Input: part model. Units: mm. Frame: model coordinates. A direction names the side the tool comes from. Coordinates: 2 decimals unless noted, no trailing zeros. Loops run counter-clockwise (first coordinate to the right, second up) from the corner with the lowest first, then second, coordinate; pieces in that order, holes last.
Item 1: Section A-A on x = -10. Return loops of the section in (y, z).
Item 2: Reachability of faces 1 (the flat face through (-16, 28.757, 4)), 2 (the flat face through (-15.383, 3.189, -0.07)), 3 (the flat face through (-1, 20, 0)) from +Z, -Z, +X, -X, +Y, -Y: full face, straight path, thin tool, end or side. Return the list, or none.
Item 3: Pull-direction query (Z, two-part tool) for faces 4 (the flat face through (4.33, 40.68, 0.06)), 5 (the flat face through (-8, 25.5, 0)), 6 (the flat face through (-16, 35, 2)); classes: released by +Z, released by -Z, zero draft, split by the parting line, or undercut.
Item 4: Ray query, line 1 along Z through (x, y) = (-10, 18.5); line 2 along Y through (x, z) = (-5.5, -2.25); line 3 along Y through (x, z) = (-8, -4.25). Return the intervals inside material, ascending.
Item 5: Contact query for flat-ended pins moving along their axis: P1, Ø3.5, axis at x = -2, z = 4, coming from the -Y side; P2, Ø2.5, axis at y = 35.5, z = -4, coming from the -X side; P3, Ø2.5, axis at x = -3, y = 35.5, coming from the -Z side; P4, Ø2, axis at x = -18, z = 2.5, coming from the +Y side. Output: stop coordinate, or through.
```python
from build123d import *

# Parameters (mm, degrees)
BOSS_EXTRUDE1_DEPTH     = 5
CUT_EXTRUDE1_DEPTH      = 52.295711322
CUT_EXTRUDE1_DEPTH_BACK = 10
CUT_EXTRUDE3_START      = -10
CUT_EXTRUDE3_DEPTH      = 10
CUT_EXTRUDE4_DEPTH      = 52.295711322
CUT_EXTRUDE4_DEPTH_BACK = 10
CUT_EXTRUDE5_DEPTH      = 10
CUT_EXTRUDE6_DEPTH      = 3
SKETCH9_R               = 4
CUT_EXTRUDE7_DEPTH      = 13
CUT_EXTRUDE8_REACH      = 41.4
SKETCH10_R              = 1.75
CUT_EXTRUDE9_DEPTH      = 13
SKETCH12_W              = 6
SKETCH12_H              = 21
CUT_EXTRUDE10_DEPTH     = 4
CUT_EXTRUDE11_DEPTH     = 5.830271703
CHAMFER1_SIZE           = 1


# Read off the part's stored shape, not the designer's step: Cut-Extrude3
with BuildPart() as part:
    # Sketch1 → Boss-Extrude1 (new, symmetric)
    with BuildSketch(Plane.XY):
        Polygon((-22.5, 45), (-22.5, 0), (22.5, 0), (22.5, 26), (3.5, 45), align=None)
    extrude(amount=BOSS_EXTRUDE1_DEPTH, both=True)

    # Sketch2 → Cut-Extrude1 (cut, two sides: drawn at the far end of the back side and taken through both)
    with BuildSketch(Plane.XY.offset(5).offset(-CUT_EXTRUDE1_DEPTH_BACK)):
        with BuildLine():
            Line((-111.960387508, -74.460387508), (-22.5, 15))
            Line((-22.5, 15), (-19.5, 18))
            Line((-19.5, 18), (-19.5, 21.5))
            ThreePointArc((-19.5, 21.5), (-17.9, 23.5), (-19.5, 25.5))
            Line((-19.5, 25.5), (-19.5, 40))
            Line((-19.5, 40), (-14.5, 45))
            Line((-14.5, 45), (74.960387508, 134.460387508))
            Line((74.960387508, 134.460387508), (-113.613392046, 303.176768247))
            Line((-113.613392046, 303.176768247), (-300.534167062, 94.255993231))
            Line((-300.534167062, 94.255993231), (-111.960387508, -74.460387508))
        make_face()
    extrude(amount=CUT_EXTRUDE1_DEPTH + CUT_EXTRUDE1_DEPTH_BACK, mode=Mode.SUBTRACT)

    # Cut-Extrude3 outline → Cut-Extrude3 (cut)
    with BuildSketch(Plane.XY.offset(5).offset(CUT_EXTRUDE3_START)):
        Polygon((21.5, 27), (21.5, 14.5), (22.5, 13.5), (22.5, 26), align=None)
        with BuildLine():
            Line((22.5, 0), (22.5, 3.8))
            ThreePointArc((22.5, 3.8), (21.972792206, 2.527207794), (20.7, 2))
            Line((20.7, 2), (17.5, 2))
            ThreePointArc((17.5, 2), (15.514097811, 3.762950432), (17.029242744, 5.943807502))
            Line((17.029242744, 5.943807502), (18.5, 6.3))
            Line((18.5, 6.3), (18.5, 7))
            Line((18.5, 7), (-16.5, 7))
            Line((-16.5, 7), (-16.5, 5.5))
            Line((-16.5, 5.5), (-15.081081244, 5.5))
            ThreePointArc((-15.081081244, 5.5), (-14.751598645, 5.326806563), (-14.707437165, 4.957206084))
            Line((-14.707437165, 4.957206084), (-16.078389668, 1.369880369))
            ThreePointArc((-16.078389668, 1.369880369), (-16.706486271, 0.552810765), (-17.679866918, 0.214228137))
            Line((-17.679866918, 0.214228137), (-21.455599386, 0.046417805))
            ThreePointArc((-21.455599386, 0.046417805), (-22.191230564, 0.322797329), (-22.5, 1.045431612))
            Line((-22.5, 1.045431612), (-22.5, 0))
            Line((-22.5, 0), (22.5, 0))
        make_face()
    extrude(amount=CUT_EXTRUDE3_DEPTH, mode=Mode.SUBTRACT)

    # Sketch3 → Cut-Extrude4 (cut, two sides: drawn at the far end of the back side and taken through both)
    with BuildSketch(Plane.XY.offset(5).offset(-CUT_EXTRUDE4_DEPTH_BACK)):
        Polygon((85.857284299, 122.40753683), (5.974873734, 42.525126266), (5.621320344, 42.171572875), (20.792893219, 27), (21.146446609, 27.353553391), (101.028857174, 107.235963955), (260.793678303, 267.000785084), (245.622105428, 282.17235796), align=None)
    extrude(amount=CUT_EXTRUDE4_DEPTH + CUT_EXTRUDE4_DEPTH_BACK, mode=Mode.SUBTRACT)

    # Sketch7 → Cut-Extrude5 (cut)
    with BuildSketch(Plane.XY.offset(5)):
        with BuildLine():
            Line((-16.5, 7.7), (-16.5, 11))
            ThreePointArc((-16.5, 11), (-16.153059775, 12.400454865), (-15.192484115, 13.476993646))
            Line((-15.192484115, 13.476993646), (-11.5, 16))
            Line((-11.5, 16), (-4.3, 16))
            ThreePointArc((-4.3, 16), (-3.734314575, 16.234314575), (-3.5, 16.8))
            Line((-3.5, 16.8), (-3.5, 22.2))
            ThreePointArc((-3.5, 22.2), (-3.734314575, 22.765685425), (-4.3, 23))
            Line((-4.3, 23), (-14.25, 23))
            ThreePointArc((-14.25, 23), (-15.5, 24.25), (-14.25, 25.5))
            Line((-14.25, 25.5), (-4.2, 25.5))
            ThreePointArc((-4.2, 25.5), (-1.9372583, 24.5627417), (-1, 22.3))
            Line((-1, 22.3), (-1, 17.183557492))
            ThreePointArc((-1, 17.183557492), (-1.825475903, 15.038415232), (-3.876022072, 14))
            Line((-3.876022072, 14), (-13.702486205, 13))
            ThreePointArc((-13.702486205, 13), (-14.98407756, 12.35099048), (-15.5, 11.010276568))
            Line((-15.5, 11.010276568), (-15.5, 7.9))
            Line((-15.5, 7.9), (-16.5, 7.7))
        make_face()
    extrude(amount=-CUT_EXTRUDE5_DEPTH, mode=Mode.SUBTRACT)

    # Sketch8 → Cut-Extrude6 (cut)
    with BuildSketch(Plane.XY.offset(5)):
        Polygon((-17.5, 20), (-13.5, 20), (-13.5, 17), (-17.5, 15), align=None)
        Polygon((-16.5, 38.757359313), (-16.5, 28.757359313), (-14.5, 28.757359313), (-14.5, 40.757359313), align=None)
        Polygon((0.4, 42), (-4.5, 42), (-4.5, 33.5), (0.4, 38.4), align=None)
        with BuildLine():
            Line((-3.52075849, 10), (18.5, 10))
            Line((18.5, 10), (18.5, 20.807611845))
            Line((18.5, 20.807611845), (16.520101013, 22.787510832))
            Line((16.520101013, 22.787510832), (8.74192642, 15.009336239))
            Line((8.74192642, 15.009336239), (4.145732342, 19.605530317))
            Line((4.145732342, 19.605530317), (11.923906935, 27.38370491))
            Line((11.923906935, 27.38370491), (6.267052685, 33.040559159))
            Line((6.267052685, 33.040559159), (0.045175397, 26.818681871))
            ThreePointArc((0.045175397, 26.818681871), (1.490346539, 24.761697843), (2, 22.3))
            Line((2, 22.3), (2, 17.183557492))
            ThreePointArc((2, 17.183557492), (0.400640437, 13.027344363), (-3.572292764, 11.015414852))
            ThreePointArc((-3.572292764, 11.015414852), (-4.029119362, 10.483214857), (-3.52075849, 10))
        make_face()
    cut_extrude6 = extrude(amount=-CUT_EXTRUDE6_DEPTH, mode=Mode.SUBTRACT)

    # Mirror1: Cut-Extrude6 across plane
    add(cut_extrude6.mirror(Plane.XY), mode=Mode.SUBTRACT)

    # Sketch9 → Cut-Extrude7 (cut)
    with BuildSketch(Plane(origin=(0, 45, 0), x_dir=(1, 0, 0), z_dir=(0, 1, 0))):
        with Locations(Location((-10, 0, 0), (0, 0, 270))):
            Circle(SKETCH9_R)
    extrude(amount=-CUT_EXTRUDE7_DEPTH, mode=Mode.SUBTRACT)

    # Cut-Extrude8: up to this face of the body (flat: up to its plane)
    cut_extrude8_end = Plane(part.part.faces().sort_by_distance((-7.9, 16, 0))[0])
    # Sketch10 → Cut-Extrude8 (cut, up to the picked face)
    with BuildSketch(Plane(origin=(0, 32, 0), x_dir=(1, 0, 0), z_dir=(0, 1, 0)), mode=Mode.PRIVATE) as cut_extrude8_sk1:
        with Locations(Location((-10, 0, 0), (0, 0, 270))):
            Circle(SKETCH10_R)
    cut_extrude8_tool1 = split(extrude(cut_extrude8_sk1.sketch, amount=-CUT_EXTRUDE8_REACH, mode=Mode.PRIVATE), bisect_by=cut_extrude8_end, keep=Keep.BOTH, mode=Mode.PRIVATE)
    add(cut_extrude8_tool1.solids().sort_by(Axis((-10, 32, 0), (0, -1, 0)))[0], mode=Mode.SUBTRACT)

    # Sketch11 → Cut-Extrude9 (cut)
    with BuildSketch(Plane.XY.offset(5)):
        with BuildLine():
            Line((-4.219533003, 31.039254845), (-0.683999097, 27.503720939))
            Line((-0.683999097, 27.503720939), (2.851534809, 31.039254845))
            Line((2.851534809, 31.039254845), (-0.683999097, 34.574788751))
            Line((-0.683999097, 34.574788751), (-2.098212659, 33.160575189))
            ThreePointArc((-2.098212659, 33.160575189), (-2.098212659, 32.453468408), (-2.80531944, 32.453468408))
            Line((-2.80531944, 32.453468408), (-4.219533003, 31.039254845))
        make_face()
        with BuildLine():
            Line((11.336816184, 18.311332784), (9.922602621, 16.897119222))
            Line((9.922602621, 16.897119222), (6.387068715, 20.432653128))
            Line((6.387068715, 20.432653128), (9.922602621, 23.968187033))
            Line((9.922602621, 23.968187033), (13.458136527, 20.432653128))
            Line((13.458136527, 20.432653128), (12.043922965, 19.018439565))
            ThreePointArc((12.043922965, 19.018439565), (11.336816184, 19.018439565), (11.336816184, 18.311332784))
        make_face()
    extrude(amount=-CUT_EXTRUDE9_DEPTH, mode=Mode.SUBTRACT)

    # Sketch12 → Cut-Extrude10 (cut)
    with BuildSketch(Plane(origin=(23.896446609, 23.896446609, 0), x_dir=(0, 0, -1), z_dir=(0.7071067811865471, 0.7071067811865479, 0))):
        with Locations((0, 15.204222165)):
            Rectangle(SKETCH12_W, SKETCH12_H)
    extrude(amount=-CUT_EXTRUDE10_DEPTH, mode=Mode.SUBTRACT)

    # Sketch13 → Cut-Extrude11 (cut)
    with BuildSketch(Plane(origin=(21.068019485, 21.068019485, 0), x_dir=(0, 0, -1), z_dir=(0.7071067811865471, 0.7071067811865479, 0))):
        Polygon((-1.5, 24.931727984), (1.5, 24.931727984), (1.5, 21.431727984), (2.75, 21.431727984), (2.75, 19.931727984), (-2.75, 19.931727984), (-2.75, 21.431727984), (-1.5, 21.431727984), align=None)
        Polygon((-1.5, 5.476716347), (-1.5, 8.976716347), (-2.75, 8.976716347), (-2.75, 10.476716347), (2.75, 10.476716347), (2.75, 8.976716347), (1.5, 8.976716347), (1.5, 5.476716347), align=None)
    extrude(amount=-CUT_EXTRUDE11_DEPTH, mode=Mode.SUBTRACT)

    # Chamfer1
    chamfer1_edges = [part.edges().sort_by_distance(p)[0] for p in [
        (13.145438014, 34.647455205, -3),
        (13.145438014, 34.647455205, 3),
    ]]
    chamfer(chamfer1_edges, length=CHAMFER1_SIZE)


solid = part.part
```
Results found:
1. outline: (7, -5) - (13.38, -5) - (13.38, 5) - (7, 5) - close; (16, -5) - (23, -5) - (23, -1.75) - (16, -1.75) - close; (16, 1.75) - (23, 1.75) - (23, 5) - (16, 5) - close; (25.5, -5) - (45, -5) - (45, -4) - (32, -4) - (32, -1.75) - (25.5, -1.75) - close; (25.5, 1.75) - (32, 1.75) - (32, 4) - (45, 4) - (45, 5) - (25.5, 5) - close
2. face 1: +Z
2. face 2: +Z, -Z, -Y
2. face 3: +Z, -Z
3. face 4: undercut
3. face 5: zero draft
3. face 6: released by +Z
4. line 1: z = -5 to -1.75, 1.75 to 5
4. line 2: y = 7 to 13.83, 16 to 23, 25.5 to 45
4. line 3: y = 7 to 13.58, 16 to 23, 25.5 to 45
5. P1: stops at y = 7
5. P2: stops at x = -19.5
5. P3: stops at z = -5
5. P4: stops at y = 42.5
